Check sheet for the modelled part. Datum: model origin and axes. Units: mm. Face numbers are marked on the shaded views. A direction names the side the tool comes from. Give positions to 0.01 mm unless a question says otherwise; leave off trailing zeros. Write each loop counter-clockwise with the first axis right and the second up, starting at its lowest first coordinate (ties: lowest second). Pieces come first, ordered by that corner, then holes. Notation, with made-up numbers: (76.25, -11) -> (135.25, -11) arc R7 cw to (135.25, -5) -> close; hole circle Ø3 at (33.25, -4.5). An arc over 180 degrees is marked (long way). Use a Markdown table: item, result. Add a question column.
1. Release check for a two-part mould opening along Y. For the marked faces 1, 2 and 3 record: released by +Y, released by -Y, zero draft, split by the parting line, or undercut.
2. Cross-section at B-B (x = 10.5). Count the separate pieces of the cut face and the enclosed holes in it, then the cut area to 3 significant figures.
3. Gauge pin test, flat ends, axial feed: P1, Ø10, axis at y = -13, z = 13, coming from the +X side; P2, Ø1, axis at y = 56.5, z = 11, coming from the +X side; P3, Ø13.5, axis at y = 71.5, z = 8, coming from the -X side; P4, Ø3, axis at y = 2, z = 26.5, coming from the -X side. Record the tip position at first contact, or that the pin passes through.
4. Cross-section at C-C (y = 69.5). Enter the section's corners in (x, z).
5. Scan lines: probe 1 along Z at (x, y) = (11, 2); probe 2 along Z at (x, y) = (1.25, 24); probe 3 along Y at (x, z) = (7.5, 26.25). Record each from-to range of solid material in increasing order. Write a range as [from, to].
6. Cross-section at A-A (y = 24). Enter the section's corners in (x, z).
7. Cross-section at D-D (x = 16.25). Enter the section's corners in (y, z), then the cut area to 3 significant figures.
8. Set-up check for the marked faces 4, 5 and 6: record each of +Z, -Z, +X, -X, +Y, -Y from which the full face is reachable in a straight line by a thin tool's end or side.
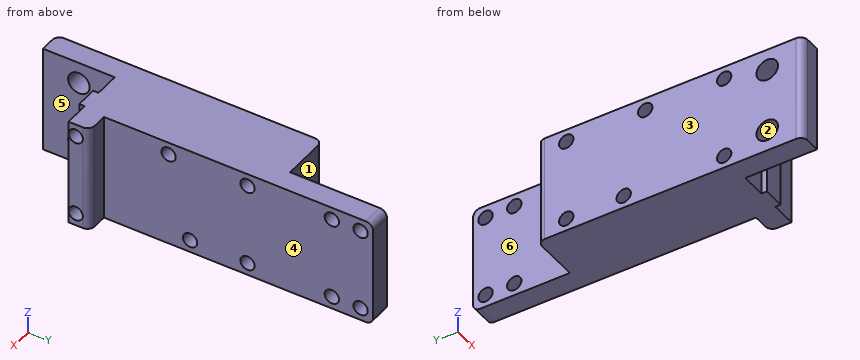
Autodesk Inventor part; units mm, degrees
ref_plane "YZ Plane" through (0, 0, 0) normal (1, 0, 0) x (0, 1, 0)
ref_plane "XZ Plane" through (0, 0, 0) normal (0, 1, 0) x (-1, 0, 0)
ref_plane "XY Plane" through (0, 0, 0) normal (0, 0, 1) x (1, 0, 0)
sketch "Sketch1" plane through (0, 0, 0) normal (0, 0, 1) x (1, 0, 0)
  line L0 (0, 0) -> (20, 0)
  line L1 (0, 0) -> (0, -20)
  line L2 (14, 6) -> (20, 6)
  line L3 (0, -20) -> (-6, -20)
  line L4 (20, 6) -> (20, 0)
  line L5 (-6, -20) -> (-6, 54)
  line L6 (14, 6) -> (14, 81)
  line L7 (8, 54) -> (8, 81)
  line L8 (8, 81) -> (14, 81)
  line L9 (8, 54) -> (-6, 54)
  dimension "d1" = 20
  dimension "d3" = 20
  dimension "d7" = 20
  dimension "d8" = 14
  dimension "d9" = 27
  dimension "d46" = 54
extrude "Extrusion1" add sketch "Sketch1" along normal blind 30
sketch "Sketch2" plane through (14, 6, 0) normal (1, 0, 0) x (0, 0, -1)
  line L0 (0, 75) -> (-30, 75)
  line L1 (-15, 75) -> (-15, 48)
  line L2 (0, 48) -> (-30, 48)
  line L3 (-30, 0) -> (-30, 75)
  line L4 (0, 0) -> (0, 75)
  line L5 (-30, 67.5) -> (0, 67.5)
  point P0 (0, -6)
  point P1 (-26.5, 71.5)
  point P2 (-3.5, 71.5)
  point P3 (-26.5, 63.5)
  point P4 (-3.5, 63.5)
  dimension "d12" = 3.5
  dimension "d13" = 3.5
hole "Hole1" at (14, 77.5, 26.5) at (14, 77.5, 3.5) at (14, 69.5, 26.5) at (14, 69.5, 3.5) direction (-1, 0, 0) diameter 4 end through all
sketch "Sketch3" plane through (0, 0, 0) normal (0, -1, 0) x (1, 0, 0)
  line L0 (0, 30) -> (20, 30)
  line L1 (0, 0) -> (20, 0)
  line L2 (13, 30) -> (13, 0)
  line L3 (7, 30) -> (7, 0)
  line L4 (13, 0) -> (7, 0)
  line L5 (7, 30) -> (13, 30)
extrude "Extrusion2" add sketch "Sketch3" along normal blind 1.5
sketch "Sketch5" plane through (-6, -20, 0) normal (-1, 0, 0) x (0, 0, 1)
  line L0 (0, 74) -> (30, 74)
  line L1 (15, 74) -> (15, 0)
  line L2 (0, 0) -> (30, 0)
  line L3 (0, 74) -> (0, 0)
  line L4 (15, 44) -> (30, 44)
  line L5 (30, 26) -> (30, 101)
  point P0 (0, 20)
  point P1 (3.5, 66)
  point P2 (26.5, 66)
  point P3 (3.5, 22)
  point P4 (26.5, 22)
  point P5 (3.5, 50)
  point P6 (26.5, 44)
  dimension "d26" = 8
  dimension "d27" = 3.5
  dimension "d28" = 30
hole "Hole2" at (-6, 46, 3.5) at (-6, 46, 26.5) at (-6, 2, 3.5) at (-6, 2, 26.5) at (-6, 30, 3.5) at (-6, 24, 26.5) direction (1, 0, 0) diameter 4 end through all
sketch "Sketch6" plane through (-6, -20, 0) normal (-1, 0, 0) x (0, 0, 1)
  line L0 (0, 0) -> (30, 0)
  line L1 (0, 74) -> (0, 0)
  line L2 (15, 0) -> (15, 31.0805)
  point P0 (0, 20)
  point P1 (6, 10)
  point P2 (24, 10)
  dimension "d36" = 10
  dimension "d37" = 6
hole "Hole3" at (-6, -10, 6) at (-6, -10, 24) direction (1, 0, 0) diameter 6 end through all
fillet "Fillet2" radius 2 5 edges at (-6, -20, 15) (20, 6, 15) (-6, 54, 15) (11, 81, 30) (11, 81, 0)
properties part number "Esteira - estrutura"
Worked answers:
| question | item | result |
|---|---|---|
| 1 | face 1 | released by +Y |
| 1 | face 2 | undercut |
| 1 | face 3 | zero draft |
| 2 | separate pieces | 1 |
| 2 | enclosed holes | 10 |
| 2 | area | 2,350 mm² |
| 3 | P1 | stops at x = 0 |
| 3 | P2 | stops at x = 14 |
| 3 | P3 | stops at x = 8 |
| 3 | P4 | passes through |
| 4 | outline | (8, 0) -> (14, 0) -> (14, 1.5) -> (8, 1.5) -> close; (8, 5.5) -> (14, 5.5) -> (14, 24.5) -> (8, 24.5) -> close; (8, 28.5) -> (14, 28.5) -> (14, 30) -> (8, 30) -> close |
| 5 | probe 1 | z = [0, 1.5], [5.5, 24.5], [28.5, 30] |
| 5 | probe 2 | z = [0, 24.5], [28.5, 30] |
| 5 | probe 3 | y = [-1.5, 0.02], [3.98, 22.02], [25.98, 44.02], [47.98, 54] |
| 6 | outline | (-6, 0) -> (14, 0) -> (14, 24.5) -> (-6, 24.5) -> close; (-6, 28.5) -> (14, 28.5) -> (14, 30) -> (-6, 30) -> close |
| 7 | outline | (0, 0) -> (6, 0) -> (6, 30) -> (0, 30) -> close; hole circle Ø4 at (2, 3.5); hole circle Ø4 at (2, 26.5) |
| 7 | area | 155 mm² |
| 8 | face 4 | +Z, -Z, +X, +Y |
| 8 | face 5 | +Z, -Z, -Y |
| 8 | face 6 | +Z, -Z, -X, +Y |
